```python
from build123d import *

# Parameters (mm, degrees)
BOSS_EXTRUDE1_DEPTH = 3
SKETCH2_W           = 3
SKETCH2_H           = 3
SKETCH2_H_2         = 36.5
SKETCH2_W_2         = 36.5
SKETCH2_W_3         = 29
SKETCH2_H_3         = 29
CUT_EXTRUDE2_DEPTH  = 3


with BuildPart() as part:
    # Sketch1 → Boss-Extrude1 (new body)
    with BuildSketch(Plane(origin=(0, 0, 0), x_dir=(1, 0, 0), z_dir=(0, 1, 0))):
        Polygon((70, 70), (-70, 70), (0, 0), align=None)
        Polygon((0, 0), (-70, 70), (-70, -70), align=None)
        Polygon((70, -70), (0, 0), (-70, -70), align=None)
        Polygon((70, 70), (0, 0), (70, -70), align=None)
    extrude(amount=BOSS_EXTRUDE1_DEPTH)

    # Sketch2 → Cut-Extrude2 (cut)
    with BuildSketch(Plane(origin=(0, 3, 0), x_dir=(1, 0, 0), z_dir=(0, 1, 0))):
        with Locations((-68.5, 68.5)):
            Rectangle(SKETCH2_W, SKETCH2_H)
        with Locations((-68.5, 48.75)):
            Rectangle(SKETCH2_W, SKETCH2_H_2)
        with Locations((-48.75, 68.5)):
            Rectangle(SKETCH2_W_2, SKETCH2_H)
        with Locations((48.75, 68.5)):
            Rectangle(SKETCH2_W_2, SKETCH2_H)
        with Locations((68.5, 68.5)):
            Rectangle(SKETCH2_W, SKETCH2_H)
        with Locations((68.5, 48.75)):
            Rectangle(SKETCH2_W, SKETCH2_H_2)
        with Locations((68.5, -68.5)):
            Rectangle(SKETCH2_W, SKETCH2_H)
        with Locations((68.5, -48.75)):
            Rectangle(SKETCH2_W, SKETCH2_H_2)
        with Locations((48.75, -68.5)):
            Rectangle(SKETCH2_W_2, SKETCH2_H)
        with Locations((-48.75, -68.5)):
            Rectangle(SKETCH2_W_2, SKETCH2_H)
        with Locations((-68.5, -68.5)):
            Rectangle(SKETCH2_W, SKETCH2_H)
        with Locations((-68.5, -48.75)):
            Rectangle(SKETCH2_W, SKETCH2_H_2)
        with Locations((0, 68.5)):
            Rectangle(SKETCH2_W_3, SKETCH2_H)
        with Locations((0, -68.5)):
            Rectangle(SKETCH2_W_3, SKETCH2_H)
        with Locations((68.5, 0)):
            Rectangle(SKETCH2_W, SKETCH2_H_3)
        with Locations((-68.5, 0)):
            Rectangle(SKETCH2_W, SKETCH2_H_3)
    extrude(amount=-CUT_EXTRUDE2_DEPTH, mode=Mode.SUBTRACT)


solid = part.part
```
Geometry check sheet. Reference: the model listing, model coordinates, mm. A direction names the side the tool comes from. Coordinates: 2 decimals unless noted, no trailing zeros. Loops run counter-clockwise (first coordinate to the right, second up) from the corner with the lowest first, then second, coordinate; pieces in that order, holes last.
Item 1: Access from +Z, -Z, +X, -X, +Y, -Y to the whole of each face (thin tool, end or side, straight path). Record for faces 1 (the face through (-69, 2, 14.5)), 2 (the face through (67, 2, 0)), 3 (the face through (-48, 2, 67)), 4 (the face through (-49, 2, -67)).
Item 2: Go/stop test with flat-tipped pins: pin 1 Ø1.5 at (x, y) = (-68, 2) entering from +Z; pin 2 Ø0.9 at (x, y) = (53.5, 1) entering from -Z; pin 3 Ø1.5 at (y, z) = (1, -68.5) entering from -X. Record where each tip stops, or that it passes through.
Item 3: Release check for a two-part mould opening along X. For faces 5 (the face through (0, 2, -67)), 6 (the face through (68, 2, -30.5)), 7 (the face through (-30.5, 2, 69)), 8 (the face through (67, 2, 48)) record: released by +X, released by -X, zero draft, split by the parting line, or undercut.
Item 4: Thickness scan on line 1 (Z direction, x = 47.5, y = 1.6). Record the ranges inside material, lowest first.
Item 5: Sectioned sample at A-A, the plane z = 1.5. Record the boundary of the cut face in (x, y).
Item 6: Sectioned sample at B-B, the plane x = -39. Record the boundary of the cut face in (y, z), then the cut area to 3 significant figures.
Check result:
1. face 1: -X, +Y, -Y
1. face 2: +X, +Y, -Y
1. face 3: +Z, -X, +Y, -Y
1. face 4: -Z, -X, +Y, -Y
2. pin 1: stops at z = 30.5
2. pin 2: stops at z = -67
2. pin 3: stops at x = -30.5
3. face 5: undercut
3. face 6: zero draft
3. face 7: released by -X
3. face 8: released by +X
4. line 1: z = -67 to 67
5. outline: (-67, 0) - (67, 0) - (67, 3) - (-67, 3) - close
6. outline: (0, -67) - (3, -67) - (3, 67) - (0, 67) - close
6. area: 402 mm2
